Could you check a few things on this model? Use its own coordinates, in mm. A direction names the side the tool comes from. Give positions to 0.01 mm unless a question says otherwise; leave off trailing zeros. Order: outer loops, then holes, each group sorted by start corner. A loop starts at its lowest first (then second) coordinate and runs counter-clockwise, first axis right, second up.
(1) Imagine slicing it at C-C, the plane y = 29. State how many separate pieces and enclosed holes the cut face has, then the cut area to 3 significant figures.
(2) If I drill on probe 1 along X at (y, z) = (3, 0); probe 2 along X at (y, z) = (13, 0), over which ranges is the centre line in solid material (lowest first)?
(3) Imagine slicing it at B-B, the plane y = 21. Write out the boundary of the cut face in (x, z) (1 decimal).
(4) On a 3-axis mill with a long thin cutter (end or side, diameter ignored), from which of +Z, -Z, +X, -X, +Y, -Y can I reach the whole of each face in a straight line? I mean faces 1 (the cylindrical face through (1.707, 17.404, 7.687)), 2 (the cylindrical face through (10.551, 31.228, -9.247)), 3 (the cylindrical face through (10.871, 3.803, -9.303)). Say none if no direction works.
(5) Imagine slicing it at D-D, the plane z = 7. Write out the boundary of the cut face in (x, y) (3 decimals), then the cut area to 3 significant figures.
(6) If we mould it in two halves opening along Z, with no side actions, what happens to faces 4 (the flat face through (8, 0, 8)), 5 (the cylindrical face through (8.6, 17.27, 16.535)), 6 (the cylindrical face through (10.551, 3.803, 9.247))? For each: released by +Z, released by -Z, zero draft, split by the parting line, or undercut.
(7) Imagine slicing it at A-A, the plane z = -6.5. Write out the boundary of the cut face in (x, y) (3 decimals).
(8) Will these pins go through, and if not, where does the flat tip stop? pin 1 (1.5 mm diameter, centred on x = 10.5, z = -10.5, fed in from +Y); pin 2 (1.5 mm diameter, centred on x = -10.5, z = 10.5, fed in from -Y); pin 3 (2 mm diameter, centred on x = 10.5, z = -10.5, fed in from +Y).
from build123d import *

# Parameters (mm, degrees)
BODY_SKETCH_R              = 18.6375
BODY_EXTRUDE_DEPTH         = 35.03125
BEARING_POCKET_SKETCH_R    = 11.049
BEARING_POCKET_CUT_1_DEPTH = 9.525
BEARING_START              = -35.03125
BEARING_POCKET_SKETCH_2_R  = 11.049
BEARING_POCKET_CUT_2_DEPTH = 9.525
BORE_SKETCH_R              = 7.874
BORE_CUT_DEPTH             = 36.03125
M3X0_5_TAPPED_HOLE1_D      = 2.5
M3X0_5_TAPPED_HOLE1_DEPTH  = 7.50062
M3X0_5_TAPPED_HOLE1_TIP    = 0.751075774
M3X0_5_TAPPED_HOLE3_D      = 2.5
M3X0_5_TAPPED_HOLE3_DEPTH  = 7.50062
M3X0_5_TAPPED_HOLE3_TIP    = 0.751075774


with BuildPart() as part:
    # Body Sketch → Body Extrude (new body)
    with BuildSketch(Plane(origin=(0, 0, 0), x_dir=(1, 0, 0), z_dir=(0, 1, 0))):
        Circle(BODY_SKETCH_R)
    extrude(amount=BODY_EXTRUDE_DEPTH)

    # Bearing Pocket Sketch → Bearing Pocket Cut 1 (cut)
    with BuildSketch(Plane(origin=(0, 0, 0), x_dir=(-1, 0, 0), z_dir=(0, -1, 0))):
        Circle(BEARING_POCKET_SKETCH_R)
    extrude(amount=-BEARING_POCKET_CUT_1_DEPTH, mode=Mode.SUBTRACT)

    # Bearing Pocket Sketch<2> → Bearing Pocket Cut 2 (cut)
    with BuildSketch(Plane(origin=(0, 0, 0), x_dir=(-1, 0, 0), z_dir=(0, -1, 0)).offset(BEARING_START)):
        Circle(BEARING_POCKET_SKETCH_2_R)
    extrude(amount=BEARING_POCKET_CUT_2_DEPTH, mode=Mode.SUBTRACT)

    # Bore Sketch → Bore Cut (cut, through all)
    with BuildSketch(Plane(origin=(0, 0, 0), x_dir=(-1, 0, 0), z_dir=(0, -1, 0))):
        Circle(BORE_SKETCH_R)
    extrude(amount=-BORE_CUT_DEPTH, mode=Mode.SUBTRACT)

    # M3x0.5 Tapped Hole1
    with Locations(Plane(origin=(0, 0, 14.843252), x_dir=(0, 0, -1), z_dir=(0, -1, 0))):
        with Locations((0, 0), (4.347487856, 10.495764144), (14.843252, 14.843252), (25.339016144, 10.495764144), (29.686504, 0), (25.339016144, -10.495764144), (14.843252, -14.843252), (4.347487856, -10.495764144)):
            Hole(M3X0_5_TAPPED_HOLE1_D / 2, depth=M3X0_5_TAPPED_HOLE1_DEPTH)
            with Locations((0, 0, -(M3X0_5_TAPPED_HOLE1_DEPTH + M3X0_5_TAPPED_HOLE1_TIP / 2))):  # 118° drill point
                Cone(0, M3X0_5_TAPPED_HOLE1_D / 2, M3X0_5_TAPPED_HOLE1_TIP, mode=Mode.SUBTRACT)

    # M3x0.5 Tapped Hole3
    with Locations(Plane(origin=(0, 35.03125, 14.843252), x_dir=(0, 0, 1), z_dir=(0, 1, 0))):
        with Locations((0, 0), (-4.347487856, 10.495764144), (-14.843252, 14.843252), (-25.339016144, 10.495764144), (-29.686504, 0), (-25.339016144, -10.495764144), (-14.843252, -14.843252), (-4.347487856, -10.495764144)):
            Hole(M3X0_5_TAPPED_HOLE3_D / 2, depth=M3X0_5_TAPPED_HOLE3_DEPTH)
            with Locations((0, 0, -(M3X0_5_TAPPED_HOLE3_DEPTH + M3X0_5_TAPPED_HOLE3_TIP / 2))):  # 118° drill point
                Cone(0, M3X0_5_TAPPED_HOLE3_D / 2, M3X0_5_TAPPED_HOLE3_TIP, mode=Mode.SUBTRACT)


solid = part.part
Answer block:
1. separate pieces: 1
1. enclosed holes: 9
1. area: 668 mm2
2. probe 1: x = -18.64 to -16.09, -13.59 to -11.05, 11.05 to 13.59, 16.09 to 18.64
2. probe 2: x = -18.64 to -7.87, 7.87 to 18.64
3. outline: circle Ø37.3 at (0, 0); hole circle Ø15.7 at (0, 0)
4. face 1: +Y, -Y
4. face 2: +Y
4. face 3: -Y
5. outline: (-17.273, 0) - (-8.549, 0) - (-8.549, 9.525) - (-3.606, 9.525) - (-3.606, 25.506) - (-8.549, 25.506) - (-8.549, 35.031) - (-17.273, 35.031) - close; (3.606, 9.525) - (8.549, 9.525) - (8.549, 0) - (17.273, 0) - (17.273, 35.031) - (8.549, 35.031) - (8.549, 25.506) - (3.606, 25.506) - close
5. area: 769 mm2
6. face 4: zero draft
6. face 5: split by the parting line
6. face 6: undercut
7. outline: (-17.467, 0) - (-8.935, 0) - (-8.935, 9.525) - (-4.444, 9.525) - (-4.444, 25.506) - (-8.935, 25.506) - (-8.935, 35.031) - (-17.467, 35.031) - close; (4.444, 9.525) - (8.935, 9.525) - (8.935, 0) - (17.467, 0) - (17.467, 35.031) - (8.935, 35.031) - (8.935, 25.506) - (4.444, 25.506) - close
8. pin 1: stops at y = 27.23
8. pin 2: stops at y = 7.8
8. pin 3: stops at y = 27.38
